Verification items for this drawing (mm, ordinates from the low corner). A direction names the side the tool comes from. Round coordinates to 2 decimals unless told otherwise and drop trailing zeros. Use a Markdown table: item, result. Add a question column.
Q1. Material ranges on L1, parallel to Z at x = 6.5, y = 12; L2, parallel to Y at x = 16, z = 2; L3, parallel to X at y = 20, z = 11.5 (1 decimal), recorded low to high.
Q2. Gauge pin test, flat ends, axial feed: P1, Ø4, axis at x = 8, z = 3, coming from the +Y side; P2, Ø1, axis at x = 9.5, y = 6, coming from the +Z side; P3, Ø5, axis at x = 24.5, z = 2.5, coming from the +Y side. Record the tip position at first contact, or that the pin passes through.
Q3. Set-up check for the marked faces 4 and 5: record each of +Z, -Z, +X, -X, +Y, -Y from which the full face is reachable in a straight line by a thin tool's end or side.
Q4. Release check for a two-part mould opening along X. For the marked faces 1, 2 and 3 record: released by +X, released by -X, zero draft, split by the parting line, or undercut.
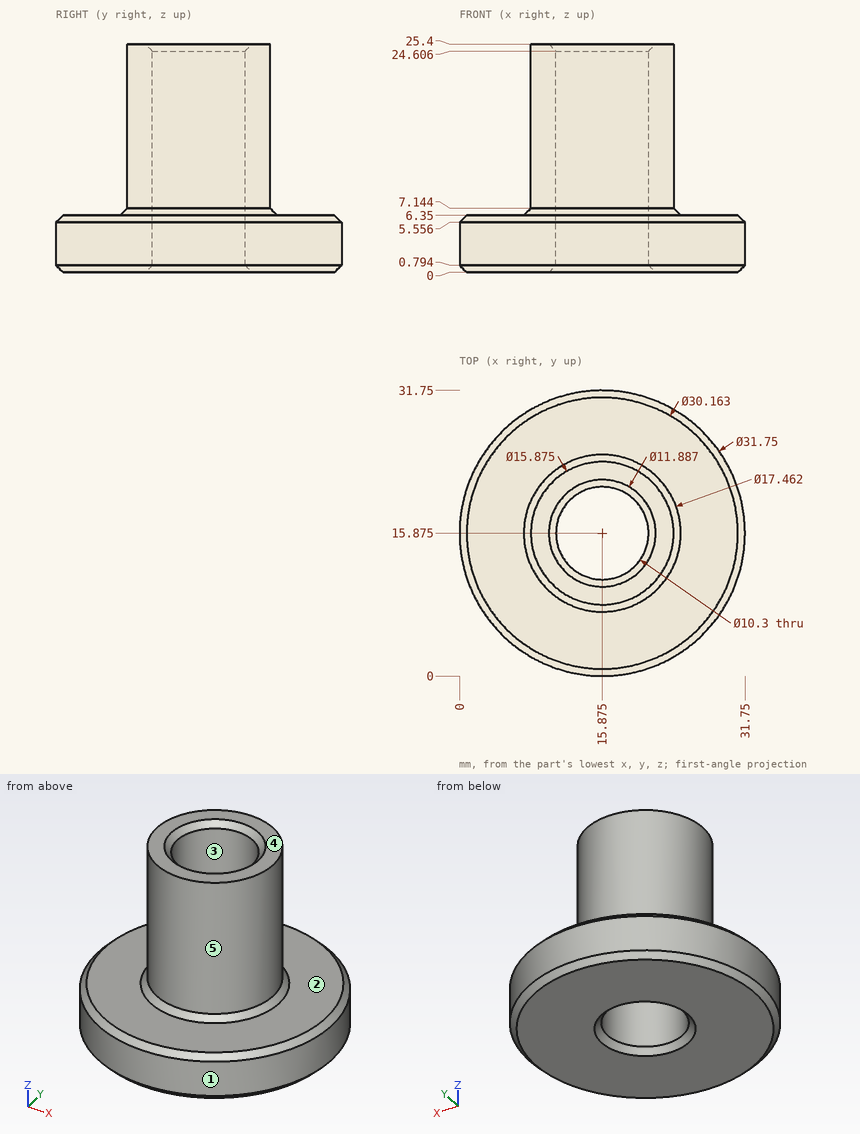
Values:
| question | item | result |
|---|---|---|
| 1 | L1 | 0 to 6.35 |
| 1 | L2 | 0 to 10.73, 21.02 to 31.75 |
| 1 | L3 | 9.1 to 12.8, 19 to 22.7 |
| 2 | P1 | y = 30.62 |
| 2 | P2 | z = 6.35 |
| 2 | P3 | y = 30.52 |
| 3 | face 4 | +Z, +X, -X, +Y, -Y |
| 3 | face 5 | +Z |
| 4 | face 1 | split by the parting line |
| 4 | face 2 | zero draft |
| 4 | face 3 | undercut |
